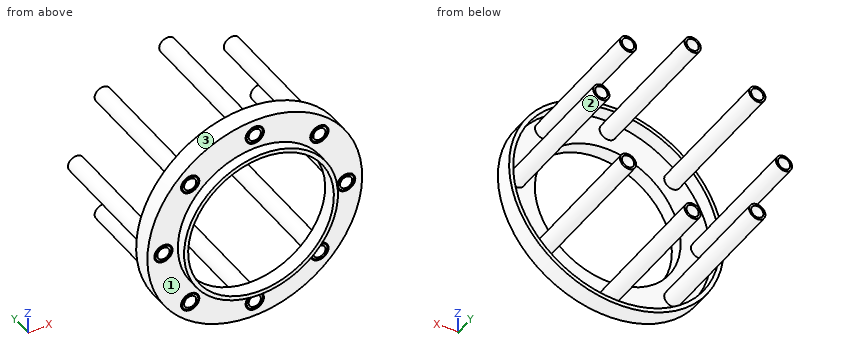
from build123d import *

# Parameters (mm, degrees)
IZIM3_R                        = 4
KES_EKSTR_ZYON1_DEPTH          = 10
PAH1_SIZE                      = 0.5
IZIM4_R                        = 4
IZIM4_R_2                      = 3
Y_KSEKLIK_EKSTR_ZYON5_DEPTH    = 70
DAIRESEL_START                 = 2.606299213
DAIRESEL_KAPLAMA15_OUTLINE_R   = 4
DAIRESEL_KAPLAMA15_OUTLINE_R_2 = 3
DAIRESEL_KAPLAMA15_DEPTH       = 68
DAIRESEL_START_2               = 0.606299213
DAIRESEL_KAPLAMA15_2_OUTLINE_R = 3
DAIRESEL_KAPLAMA15_2_DEPTH     = 2


# Read off the part's stored shape, not the designer's step: Dairesel Kaplama15
with BuildPart() as part:
    # Çizim1 → Döndür2 (revolve)
    with BuildSketch(Plane.XY, mode=Mode.PRIVATE) as d_nd_r2_sk:
        Polygon((-52.9, 9.606299213), (-52.9, 0.606299213), (-37.9, 0.606299213), (-37.9, -4.393700787), (-35.9, -4.393700787), (-35.9, 2.606299213), (-50.9, 2.606299213), (-50.9, 9.606299213), align=None)
    revolve(d_nd_r2_sk.sketch.rotate(Axis((0, 16.98519685, 0), (0, -1, 0)), 270), axis=Axis((0, 16.98519685, 0), (0, -1, 0)))

    # Çizim3 → Kes-Ekstrüzyon1 (cut)
    with BuildSketch(Plane.XZ.offset(-0.606299213)):
        with Locations(Location((0, 45, 0), (0, 0, 270))):
            Circle(IZIM3_R)
    extrude(amount=-KES_EKSTR_ZYON1_DEPTH, mode=Mode.SUBTRACT)

    # Pah1
    pah1_edges = [part.edges().sort_by_distance(p)[0] for p in [
        (0, 0.606299213, 49),
    ]]
    chamfer(pah1_edges, length=PAH1_SIZE)

    # Çizim4 → Yükseklik-Ekstrüzyon5 (add)
    with BuildSketch(Plane.XZ.offset(-0.606299213)):
        with Locations(Location((0, 45, 0), (0, 0, 270))):
            Circle(IZIM4_R)
        with Locations(Location((0, 45, 0), (0, 0, 270))):
            Circle(IZIM4_R_2, mode=Mode.SUBTRACT)
    extrude(amount=-Y_KSEKLIK_EKSTR_ZYON5_DEPTH)

    # Dairesel Kaplama15 outline → Dairesel Kaplama15 (add)
    # profile 1 of 7: a face of its own
    with BuildSketch(Plane(origin=(0, 0, 0), x_dir=(1, 0, 0), z_dir=(0, 1, 0)).offset(DAIRESEL_START)):
        with Locations((31.819805153, -31.819805153)):
            Circle(DAIRESEL_KAPLAMA15_OUTLINE_R)
        with Locations((31.819805153, -31.819805153)):
            Circle(DAIRESEL_KAPLAMA15_OUTLINE_R_2, mode=Mode.SUBTRACT)
    # profile 2 of 7: a face of its own
    with BuildSketch(Plane(origin=(0, 0, 0), x_dir=(1, 0, 0), z_dir=(0, 1, 0)).offset(DAIRESEL_START)):
        with Locations((45, 0)):
            Circle(DAIRESEL_KAPLAMA15_OUTLINE_R)
        with Locations((45, 0)):
            Circle(DAIRESEL_KAPLAMA15_OUTLINE_R_2, mode=Mode.SUBTRACT)
    # profile 3 of 7: a face of its own
    with BuildSketch(Plane(origin=(0, 0, 0), x_dir=(1, 0, 0), z_dir=(0, 1, 0)).offset(DAIRESEL_START)):
        with Locations((31.819805153, 31.819805153)):
            Circle(DAIRESEL_KAPLAMA15_OUTLINE_R)
        with Locations((31.819805153, 31.819805153)):
            Circle(DAIRESEL_KAPLAMA15_OUTLINE_R_2, mode=Mode.SUBTRACT)
    # profile 4 of 7: a face of its own
    with BuildSketch(Plane(origin=(0, 0, 0), x_dir=(1, 0, 0), z_dir=(0, 1, 0)).offset(DAIRESEL_START)):
        with Locations((0, 45)):
            Circle(DAIRESEL_KAPLAMA15_OUTLINE_R)
        with Locations((0, 45)):
            Circle(DAIRESEL_KAPLAMA15_OUTLINE_R_2, mode=Mode.SUBTRACT)
    # profile 5 of 7: a face of its own
    with BuildSketch(Plane(origin=(0, 0, 0), x_dir=(1, 0, 0), z_dir=(0, 1, 0)).offset(DAIRESEL_START)):
        with Locations((-31.819805153, 31.819805153)):
            Circle(DAIRESEL_KAPLAMA15_OUTLINE_R)
        with Locations((-31.819805153, 31.819805153)):
            Circle(DAIRESEL_KAPLAMA15_OUTLINE_R_2, mode=Mode.SUBTRACT)
    # profile 6 of 7: a face of its own
    with BuildSketch(Plane(origin=(0, 0, 0), x_dir=(1, 0, 0), z_dir=(0, 1, 0)).offset(DAIRESEL_START)):
        with Locations((-45, 0)):
            Circle(DAIRESEL_KAPLAMA15_OUTLINE_R)
        with Locations((-45, 0)):
            Circle(DAIRESEL_KAPLAMA15_OUTLINE_R_2, mode=Mode.SUBTRACT)
    # profile 7 of 7: a face of its own
    with BuildSketch(Plane(origin=(0, 0, 0), x_dir=(1, 0, 0), z_dir=(0, 1, 0)).offset(DAIRESEL_START)):
        with Locations((-31.819805153, -31.819805153)):
            Circle(DAIRESEL_KAPLAMA15_OUTLINE_R)
        with Locations((-31.819805153, -31.819805153)):
            Circle(DAIRESEL_KAPLAMA15_OUTLINE_R_2, mode=Mode.SUBTRACT)
    extrude(amount=DAIRESEL_KAPLAMA15_DEPTH)

    # Dairesel Kaplama15 2 outline → Dairesel Kaplama15 2 (cut)
    with BuildSketch(Plane(origin=(0, 0, 0), x_dir=(1, 0, 0), z_dir=(0, 1, 0)).offset(DAIRESEL_START_2)):
        with Locations((31.819805153, -31.819805153)):
            Circle(DAIRESEL_KAPLAMA15_2_OUTLINE_R)
        with Locations((45, 0)):
            Circle(DAIRESEL_KAPLAMA15_2_OUTLINE_R)
        with Locations((31.819805153, 31.819805153)):
            Circle(DAIRESEL_KAPLAMA15_2_OUTLINE_R)
        with Locations((0, 45)):
            Circle(DAIRESEL_KAPLAMA15_2_OUTLINE_R)
        with Locations((-31.819805153, 31.819805153)):
            Circle(DAIRESEL_KAPLAMA15_2_OUTLINE_R)
        with Locations((-45, 0)):
            Circle(DAIRESEL_KAPLAMA15_2_OUTLINE_R)
        with Locations((-31.819805153, -31.819805153)):
            Circle(DAIRESEL_KAPLAMA15_2_OUTLINE_R)
    extrude(amount=DAIRESEL_KAPLAMA15_2_DEPTH, mode=Mode.SUBTRACT)

    # Dairesel Kaplama15 3 outline → Dairesel Kaplama15 3 (revolve, cut)
    with BuildSketch(Plane(origin=(31.819805153, 0, 31.819805153), x_dir=(1, 0, 0), z_dir=(0, 0, 1))):
        Polygon((4.5, 0.606299213), (4, 1.106299213), (4, 0.606299213), align=None)
    revolve(axis=Axis((31.819805153, 0, 31.819805153), (0, 1, 0)), mode=Mode.SUBTRACT)

    # Dairesel Kaplama15 4 outline → Dairesel Kaplama15 4 (revolve, cut)
    with BuildSketch(Plane(origin=(45, 0, 0), x_dir=(1, 0, 0), z_dir=(0, 0, 1))):
        Polygon((4.5, 0.606299213), (4, 1.106299213), (4, 0.606299213), align=None)
    revolve(axis=Axis((45, 0, 0), (0, 1, 0)), mode=Mode.SUBTRACT)

    # Dairesel Kaplama15 5 outline → Dairesel Kaplama15 5 (revolve, cut)
    with BuildSketch(Plane(origin=(31.819805153, 0, -31.819805153), x_dir=(1, 0, 0), z_dir=(0, 0, 1))):
        Polygon((4.5, 0.606299213), (4, 1.106299213), (4, 0.606299213), align=None)
    revolve(axis=Axis((31.819805153, 0, -31.819805153), (0, 1, 0)), mode=Mode.SUBTRACT)

    # Dairesel Kaplama15 6 outline → Dairesel Kaplama15 6 (revolve, cut)
    with BuildSketch(Plane.XY.offset(-45)):
        Polygon((4.5, 0.606299213), (4, 1.106299213), (4, 0.606299213), align=None)
    revolve(axis=Axis((0, 0, -45), (0, 1, 0)), mode=Mode.SUBTRACT)

    # Dairesel Kaplama15 7 outline → Dairesel Kaplama15 7 (revolve, cut)
    with BuildSketch(Plane(origin=(-31.819805153, 0, -31.819805153), x_dir=(1, 0, 0), z_dir=(0, 0, 1))):
        Polygon((4.5, 0.606299213), (4, 1.106299213), (4, 0.606299213), align=None)
    revolve(axis=Axis((-31.819805153, 0, -31.819805153), (0, 1, 0)), mode=Mode.SUBTRACT)

    # Dairesel Kaplama15 8 outline → Dairesel Kaplama15 8 (revolve, cut)
    with BuildSketch(Plane(origin=(-45, 0, 0), x_dir=(1, 0, 0), z_dir=(0, 0, 1))):
        Polygon((4.5, 0.606299213), (4, 1.106299213), (4, 0.606299213), align=None)
    revolve(axis=Axis((-45, 0, 0), (0, 1, 0)), mode=Mode.SUBTRACT)

    # Dairesel Kaplama15 9 outline → Dairesel Kaplama15 9 (revolve, cut)
    with BuildSketch(Plane(origin=(-31.819805153, 0, 31.819805153), x_dir=(1, 0, 0), z_dir=(0, 0, 1))):
        Polygon((4.5, 0.606299213), (4, 1.106299213), (4, 0.606299213), align=None)
    revolve(axis=Axis((-31.819805153, 0, 31.819805153), (0, 1, 0)), mode=Mode.SUBTRACT)


solid = part.part
Source: CAD feature listing. Evaluate the final solid. Frame: model axes, mm. Face numbers are marked on the shaded views. Round coordinates to 2 decimals unless told otherwise and drop trailing zeros. Write each loop counter-clockwise with the first axis right and the second up, starting at its lowest first coordinate (ties: lowest second). Pieces come first, ordered by that corner, then holes. Notation, with made-up numbers: (52, -11) - (85, -11) arc R15 ccw to (85, 13) - close; hole circle Ø4 at (8.25, 18.25). An arc over 180 degrees is marked (long way). Use CSV: the item, a comma, the result in double quotes. Start each with the question number.
(1) Cut plane B-B, the plane y = 17. Give the number of separate pieces and of enclosed holes in the cut face, and give its area (3 significant figures).
(2) Mould query, pull axis X, two halves, no side actions, for the marked faces 1, 2 and 3. Classes: pulls with the +X half, pulls with the -X half, needs draft (parallel to the pull), parting line crosses it, or undercut.
(3) Cut plane A-A, the plane z = -25. Return loops of the section in (x, y).
(4) First-contact query: pin 1 Ø5 at (x, y) = (-39.5, 25) entering from +Z; pin 2 Ø4 at (x, z) = (30.5, -32) entering from -Y; pin 3 Ø10 at (y, z) = (50.5, 32.5) entering from +X; pin 4 Ø5.5 at (x, z) = (45, 0) entering from -Y. Flat tips, straight axial feed; report the tip coordinate or a pass-through.
(5) Cut plane C-C, the plane x = 45. Return loops of the section in (y, z), and give its area (3 significant figures).
(6) Material intervals for probe 1 along Z at (x, y) = (-34, 42.5); probe 2 along X at (y, z) = (4.5, -33.5); probe 3 along X at (y, z) = (39, 33), sorted ascending. Write a range as [from, to].
Geometry says:
1,separate pieces,"8"
1,enclosed holes,"8"
1,area,"176 mm²"
2,face 1,"needs draft"
2,face 2,"undercut"
2,face 3,"parting line crosses it"
3,outline,"(-46.62, 0.61) - (-28.49, 0.61) - (-28.49, -4.39) - (-25.76, -4.39) - (-25.76, 2.61) - (-44.34, 2.61) - (-44.34, 9.61) - (-46.62, 9.61) - close; (25.76, -4.39) - (28.49, -4.39) - (28.49, 0.61) - (46.62, 0.61) - (46.62, 9.61) - (44.34, 9.61) - (44.34, 2.61) - (25.76, 2.61) - close"
4,pin 1,"z = 2.65"
4,pin 2,"y = 0.61"
4,pin 3,"x = 35.82"
4,pin 4,"through"
5,outline,"(0.61, -27.81) - (9.61, -27.81) - (9.61, -23.79) - (2.61, -23.79) - (2.61, -4) - (70.61, -4) - (70.61, -3) - (0.61, -3) - (0.61, -4) - (1.11, -4) - (0.61, -4.5) - close; (0.61, 3) - (70.61, 3) - (70.61, 4) - (2.61, 4) - (2.61, 23.79) - (9.61, 23.79) - (9.61, 27.81) - (0.61, 27.81) - (0.61, 4.5) - (1.11, 4) - (0.61, 4) - close"
5,area,"291 mm²"
6,probe 1,"[-35.17, -33.88], [-29.76, -28.47], [28.47, 29.76], [33.88, 35.17]"
6,probe 2,"[-40.94, -38.32], [-35.45, -34.31], [-29.33, -28.19], [28.19, 29.33], [34.31, 35.45], [38.32, 40.94]"
6,probe 3,"[-35.64, -34.58], [-29.06, -28], [28, 29.06], [34.58, 35.64]"
